Autodesk Inventor part; units mm, degrees
ref_plane "YZ Plane" through (0, 0, 0) normal (1, 0, 0) x (0, 1, 0)
ref_plane "XZ Plane" through (0, 0, 0) normal (0, 1, 0) x (-1, 0, 0)
ref_plane "XY Plane" through (0, 0, 0) normal (0, 0, 1) x (1, 0, 0)
sketch "Sketch1" plane through (0, 0, 0) normal (0, 1, 0) x (-1, 0, 0)
  line L0 (-3.6662, 6.35) -> (3.6662, 6.35)
  line L1 (3.6662, 6.35) -> (7.3323, 0)
  line L2 (7.3323, 0) -> (3.6662, -6.35)
  line L3 (3.6662, -6.35) -> (-3.6662, -6.35)
  line L4 (-3.6662, -6.35) -> (-7.3323, 0)
  line L5 (-7.3323, 0) -> (-3.6662, 6.35)
  point P0 (0, 0)
  point P1 (0, 0)
  dimension "d0" = 12.7
extrude "Extrusion1" add sketch "Sketch1" along normal blind 42.8625
sketch "Sketch2" plane through (0, 42.8625, 0) normal (0, 1, 0) x (1, 0, 0)
  circle A0 centre (0, 0) radius 2.54
  dimension "d3" = 5.08
extrude "Extrusion2" cut sketch "Sketch2" against normal blind 25.4
thread "Thread1"
sketch "Sketch3" plane through (0, 0, 0) normal (0, -1, 0) x (1, 0, 0)
  circle A0 centre (0, 0) radius 2.54
  dimension "d8" = 5.08
extrude "Extrusion3" cut sketch "Sketch3" against normal blind 25.4
thread "Thread2"
properties part number "OUTK_016_Shaft4" material "Aluminum 6061"
Source: CAD feature listing. Evaluate the final solid. Frame: model axes, mm. Round coordinates to 2 decimals unless told otherwise and drop trailing zeros. Loops run counter-clockwise (first coordinate to the right, second up) from the corner with the lowest first, then second, coordinate; pieces in that order, holes last. Notation, with made-up numbers: M -22.5,-9.5 L 3.5,-9.5 A24 ccw 3.5,15.5 Z; hole C -10.75,39.25 d2. An arc over 180 degrees is marked long. Use a Markdown table: item, result. Add a question column.
1. Section query C-C on z = -1.5. Return the cut outline in (x, y), then the cut area to 3 significant figures.
2. Section query A-A on x = 0. Return the cut outline in (y, z).
3. Mould query, pull axis X, two halves, no side actions, for faces 1 (the flat face through (5.525, 21.131, 3.131)), 2 (the flat face through (-3, 0, 0)), 3 (the flat face through (-5.525, 21.131, -3.131)), 4 (the cylindrical face through (-0.33, 21.13, 2.52)). Classes: pulls with the +X half, pulls with the -X half, needs draft (parallel to the pull), parting line crosses it, or undercut.
4. Line query: line 1 (Z direction, x = 0, y = 16.5); line 2 (X direction, y = 10, z = 0); line 3 (X direction, y = 20, z = -0.25). Output: solid intervals per line, ascending.
5. Contact query for flat-ended pins moving along their axis: P1, Ø2, axis at y = 7, z = -2.5, coming from the +X side; P2, Ø1.5, axis at y = 6.5, z = -2.5, coming from the -X side; P3, Ø1.5, axis at x = 0.5, z = 1.5, coming from the -Y side. Output: stop coordinate, or through.
6. Section query B-B on y = 18.5. Return the cut outline in (x, z), then the cut area to 3 significant figures.
7. Section query D-D on z = 3.75. Return the cut outline in (x, y).
Reported:
| question | item | result |
|---|---|---|
| 1 | outline | M -6.47,0 L -2.05,0 L -2.05,42.86 L -6.47,42.86 Z; M 2.05,0 L 6.47,0 L 6.47,42.86 L 2.05,42.86 Z |
| 1 | area | 379 mm² |
| 2 | outline | M 0,-6.35 L 42.86,-6.35 L 42.86,-2.54 L 0,-2.54 Z; M 0,2.54 L 42.86,2.54 L 42.86,6.35 L 0,6.35 Z |
| 3 | face 1 | pulls with the +X half |
| 3 | face 2 | needs draft |
| 3 | face 3 | pulls with the -X half |
| 3 | face 4 | undercut |
| 4 | line 1 | z = -6.35 to -2.54, 2.54 to 6.35 |
| 4 | line 2 | x = -7.33 to -2.54, 2.54 to 7.33 |
| 4 | line 3 | x = -7.19 to -2.53, 2.53 to 7.19 |
| 5 | P1 | stops at x = 6.47 |
| 5 | P2 | stops at x = -6.32 |
| 5 | P3 | passes through |
| 6 | outline | M -7.33,0 L -3.67,-6.35 L 3.67,-6.35 L 7.33,0 L 3.67,6.35 L -3.67,6.35 Z; hole C 0,0 d5.08 |
| 6 | area | 119 mm² |
| 7 | outline | M -5.17,0 L 5.17,0 L 5.17,42.86 L -5.17,42.86 Z |
